```python
from build123d import *

# Parameters (mm, degrees)
EXTRUDE_1_DEPTH     = 1.5
EXTRUDE_2_DEPTH     = 5
SKETCH_5_W          = 1.4
SKETCH_5_H          = 2.6
CUT_EXTRUDE_1_DEPTH = 48.8565565


with BuildPart() as part:
    # 草图1 → 凸台-拉伸1 (new body)
    with BuildSketch(Plane.XY):
        with BuildLine():
            Line((-17, 22), (17, 22))
            ThreePointArc((17, 22), (20.535533906, 20.535533906), (22, 17))
            Line((22, 17), (22, -17))
            ThreePointArc((22, -17), (20.535533906, -20.535533906), (17, -22))
            Line((17, -22), (-17, -22))
            ThreePointArc((-17, -22), (-20.535533906, -20.535533906), (-22, -17))
            Line((-22, -17), (-22, 17))
            ThreePointArc((-22, 17), (-20.535533906, 20.535533906), (-17, 22))
        make_face()
    extrude(amount=EXTRUDE_1_DEPTH)

    # 草图2 → 凸台-拉伸2 (add)
    with BuildSketch(Plane.XY.offset(1.5)):
        with BuildLine():
            Line((-17, 22), (17, 22))
            ThreePointArc((17, 22), (20.535533906, 20.535533906), (22, 17))
            Line((22, 17), (22, -17))
            ThreePointArc((22, -17), (20.535533906, -20.535533906), (17, -22))
            Line((17, -22), (-17, -22))
            ThreePointArc((-17, -22), (-20.535533906, -20.535533906), (-22, -17))
            Line((-22, -17), (-22, 17))
            ThreePointArc((-22, 17), (-20.535533906, 20.535533906), (-17, 22))
        make_face()
        with BuildLine():
            Line((-15, 20), (15, 20))
            ThreePointArc((15, 20), (18.535533906, 18.535533906), (20, 15))
            Line((20, 15), (20, -15))
            ThreePointArc((20, -15), (18.535533906, -18.535533906), (15, -20))
            Line((15, -20), (-15, -20))
            ThreePointArc((-15, -20), (-18.535533906, -18.535533906), (-20, -15))
            Line((-20, -15), (-20, 15))
            ThreePointArc((-20, 15), (-18.535533906, 18.535533906), (-15, 20))
        make_face(mode=Mode.SUBTRACT)
    extrude(amount=EXTRUDE_2_DEPTH)

    # 草图5 → 切除-拉伸1 (cut, through all)
    with BuildSketch(Plane(origin=(-20, 0, 0), x_dir=(0, 0, -1), z_dir=(1, 0, 0))):
        with Locations((-2.2, 0)):
            Rectangle(SKETCH_5_W, SKETCH_5_H)
    extrude(amount=-CUT_EXTRUDE_1_DEPTH, mode=Mode.SUBTRACT)


solid = part.part
```
For this review, take the finished solid that the model builds, in its own axes (mm). A direction names the side the tool comes from. Give positions to 0.01 mm unless a question says otherwise; leave off trailing zeros. Write each loop counter-clockwise with the first axis right and the second up, starting at its lowest first coordinate (ties: lowest second). Pieces come first, ordered by that corner, then holes. Notation, with made-up numbers: M -1,76.5 L 9,76.5 A20 cw 9,95.5 Z; hole C 20,-1 d8. An arc over 180 degrees is marked long. Answer as a JSON object with one key per item and string values. Group by question number.
Item 1: For pin 1 Ø1.5 at (x, z) = (-21.5, 2.5) entering from +Y; pin 2 Ø2 at (x, y) = (-4.5, 0) entering from +Z; pin 3 Ø12 at (x, y) = (3, -6.5) entering from -Z; pin 4 Ø1.1 at (x, z) = (-21, 2) entering from -Y, all flat-tipped, find the tip position at first contact; note any pin that passes through.
Item 2: Draft analysis for pull direction X (two halves, no side actions). For faces 1 (the flat face through (-20, 0, 4)), 2 (the cylindrical face through (-21, 20, 3)), 3 (the flat face through (0, 22, 3)), state which applies: +X half, -X half, draft (parallel to the pull), parting line (faces both ways), or undercut.
Item 3: Consider section B-B on z = 3.75. Write out the cut boundary in (x, y), plus the area to 3 significant figures.
Item 4: Tool access review of faces 4 (the flat face through (-22, -0.2, 3.2)), 5 (the flat face through (20, 0, 4)), 6 (the flat face through (-21, -1.3, 2)): name each direction out of +Z, -Z, +X, -X, +Y, -Y from which nothing blocks a thin tool from reaching the whole face with its end or side.
Item 5: Consider section A-A on x = -13.5. Write out the cut boundary in (y, z).
Item 6: For probe 1 along Y at (x, z) = (-13, 2.75); probe 2 along Z at (x, y) = (12, -8.5), list the stretches that pass through material, from the lowest coordinate up. Write a range as [from, to].
Check result:
{
 "1": {"pin 1": "stops at y = 20.31", "pin 2": "stops at z = 1.5", "pin 3": "stops at z = 0", "pin 4": "stops at y = -20.62"},
 "2": {"face 1": "undercut", "face 2": "-X half", "face 3": "draft"},
 "3": {"outline": "M -22,-17 A5 ccw -17,-22 L 17,-22 A5 ccw 22,-17 L 22,17 A5 ccw 17,22 L -17,22 A5 ccw -22,17 Z; hole M -20,-15 A5 ccw -15,-20 L 15,-20 A5 ccw 20,-15 L 20,15 A5 ccw 15,20 L -15,20 A5 ccw -20,15 Z", "area": "336 mm^2"},
 "4": {"face 4": "+Z, -Z, -X, +Y, -Y", "face 5": "+Z", "face 6": "-X"},
 "5": {"outline": "M -22,0 L 22,0 L 22,6.5 L 20,6.5 L 20,1.5 L -20,1.5 L -20,6.5 L -22,6.5 Z"},
 "6": {"probe 1": "y = [-22, -20], [20, 22]", "probe 2": "z = [0, 1.5]"}
}
